```python
from build123d import *

# Parameters (mm, degrees)
F0_W     = 40
F0_H     = 40
F0_W_2   = 34
F0_H_2   = 34
F1_DEPTH = 250
F2_W     = 5
F2_H     = 55
F3_DEPTH = 20
F4_R     = 2.5
F5_DEPTH = 255


with BuildPart() as f1:
    # F0 (on Front) → F1 (new body, symmetric)
    with BuildSketch(Plane.XZ):
        Rectangle(F0_W, F0_H)
        Rectangle(F0_W_2, F0_H_2, mode=Mode.SUBTRACT)
    extrude(amount=F1_DEPTH, both=True)

    # F2 (on Right) → F3 (join, symmetric)
    with BuildSketch(Plane.YZ):
        with Locations((-252.5, 7.5)):
            Rectangle(F2_W, F2_H)
        with Locations((252.5, 7.5)):
            Rectangle(F2_W, F2_H)
    extrude(amount=F3_DEPTH, both=True)

    # F4 (on Front) → F5 (cut, symmetric)
    with BuildSketch(Plane.XZ):
        with Locations((-15, 30)):
            Circle(F4_R)
        with Locations((15, 30)):
            Circle(F4_R)
    extrude(amount=F5_DEPTH, both=True, mode=Mode.SUBTRACT)


solid = f1.part
```
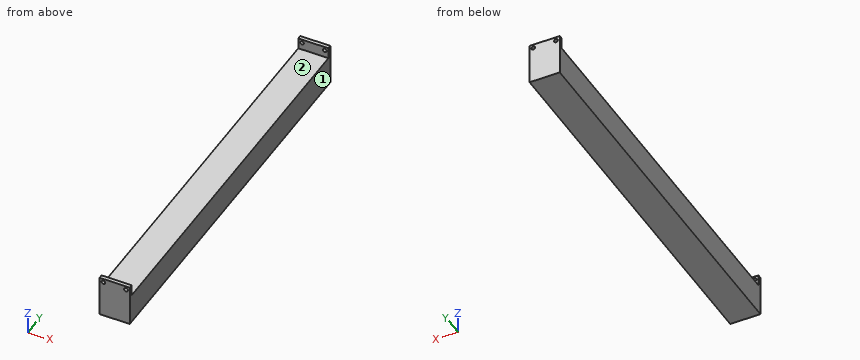
Model file for the job. Use its own axes, mm. Face numbers are marked on the shaded views. A direction names the side the tool comes from. Round coordinates to 2 decimals unless told otherwise and drop trailing zeros. Write each loop counter-clockwise with the first axis right and the second up, starting at its lowest first coordinate (ties: lowest second). Pieces come first, ordered by that corner, then holes. Notation, with made-up numbers: (60, 17) - (99, 17) arc R13 ccw to (99, 29) - close; hole circle Ø9 at (-27.5, 34.25). An arc over 180 degrees is marked (long way). One line per item, written item: value.
(1) 3-axis set-ups, long thin cutter, end or side, ignore diameter. For the marked faces 1 and 2: which of +Z, -Z, +X, -X, +Y, -Y reach the whole face in a straight line?
Values follow:
face 1: +Z, -Z, +X, +Y, -Y
face 2: +Z, +X, -X
(2) Cut at C-C, the plane y = -172. Give the cut face in (x, z), plus the area to 3 significant figures.
Values follow:
outline: (-20, -20) - (20, -20) - (20, 20) - (-20, 20) - close; hole (-17, -17) - (17, -17) - (17, 17) - (-17, 17) - close
area: 444 mm²
(3) Cut at B-B, the plane x = 8. Give the cut face in (y, z).
Values follow:
outline: (-255, -20) - (255, -20) - (255, 35) - (250, 35) - (250, 20) - (-250, 20) - (-250, 35) - (-255, 35) - close; hole (-250, -17) - (250, -17) - (250, 17) - (-250, 17) - close
(4) Drop a flat-ended pin along its axis: P1, Ø10, axis at x = 9.5, y = -74.5, coming from the +Z side. Give the stop position or say it passes through.
Values follow:
P1: stops at z = 20
(5) Wall check: probe 1 along Z at (x, y) = (-5.5, 43); probe 2 along Y at (x, z) = (16.5, 24). Give the ranges that are in metal, low to high.
Values follow:
probe 1: z = -20 to -17, 17 to 20
probe 2: y = -255 to -250, 250 to 255
(6) Cut at A-A, the plane z = -1. Give the cut face in (x, y), plus the area to 3 significant figures.
Values follow:
outline: (-20, -255) - (20, -255) - (20, 255) - (-20, 255) - close; hole (-17, -250) - (17, -250) - (17, 250) - (-17, 250) - close
area: 3,400 mm²
